Model file for the job. Use its own axes, mm. A direction names the side the tool comes from. Give positions to 0.01 mm unless a question says otherwise; leave off trailing zeros. Order: outer loops, then holes, each group sorted by start corner. A loop starts at its lowest first (then second) coordinate and runs counter-clockwise, first axis right, second up. Notation, with made-up numbers: (84, 30.25) -> (125, 30.25) arc R14 ccw to (125, 57.25) -> close; hole circle Ø3 at (58, 18). An arc over 180 degrees is marked (long way). Use CSV: the item, a comma, the result in double quotes. Start each with the question number.
1. Cut at B-B on z = 1.75. Give the number of separate pieces and of enclosed holes in the cut face, then the cut area to 3 significant figures.
2. Wall check: line 1 (X direction, y = 14.5, z = 11.5); line 2 (X direction, y = 1.25, z = -15.75); line 3 (X direction, y = 2.15, z = 19.75). Give the ranges that are in metal, low to high. Write a range as from..to.
3. Cut at C-C on z = 12.5. List the corners of the cut face in (x, y), then the cut area to 3 significant figures.
4. Drop flat-ended pins along their axis: pin 1 (18 mm diameter, centred on x = -1, z = 4.5, fed in from +Y); pin 2 (6 mm diameter, centred on y = 8, z = -17, fed in from +X); pin 3 (3 mm diameter, centred on y = 11.5, z = -7, fed in from -X); pin 4 (1 mm diameter, centred on x = -30.5, z = -3, fed in from -Y). Give the stop position or say it passes through.
5. Pull direction Z, two halves, no side cores. Call faces 4 (the flat face through (-70, 16, 0)), 5 (the cylindrical face through (-72.297, 6.535, -32.609)), 6 (the flat face through (16, 2, 8.25)): released by +Z, released by -Z, zero draft, split by the parting line, or undercut.
6. 3-axis set-ups, long thin cutter, end or side, ignore diameter. For faces 1 (the flat face through (-44.295, 2, 12)), 2 (the flat face through (-73.5, 9, 0)), 3 (the cylindrical face through (-73.609, 2.028, -33.797)): which of +Z, -Z, +X, -X, +Y, -Y reach the whole face in a straight line?
7. Cut at A-A on z = 19.75. List the corners of the cut face in (x, y).
```python
from build123d import *

# Parameters (mm, degrees)
SKETCH1_W           = 149.5
SKETCH1_H           = 70
BOSS_EXTRUDE1_DEPTH = 4
FILLET1_R           = 4
SKETCH6_W           = 147
SKETCH6_H           = 67.5
BOSS_EXTRUDE3_DEPTH = 5
FILLET2_R           = 4
SKETCH7_W           = 6.205469591
SKETCH7_H           = 30
BOSS_EXTRUDE4_DEPTH = 7
SKETCH8_R           = 1
CUT_EXTRUDE3_DEPTH  = 154.163515564
FILLET5_R           = 4
SKETCH9_W           = 134.589060818
SKETCH9_H           = 59.5
CUT_EXTRUDE4_DEPTH  = 5
FILLET7_R           = 2
SKETCH11_R          = 4
CUT_EXTRUDE5_DEPTH  = 84.406009975
SKETCH12_R          = 2.75
CUT_EXTRUDE6_DEPTH  = 84.406009975
SKETCH13_R          = 2.75
CUT_EXTRUDE7_DEPTH  = 84.406009975
SKETCH17_W          = 16
SKETCH17_H          = 13
CUT_EXTRUDE11_DEPTH = 84.406009975
SKETCH18_R          = 3
SKETCH18_W          = 15
SKETCH18_H          = 7
CUT_EXTRUDE12_DEPTH = 84.406009975
SKETCH19_W          = 6
SKETCH19_H          = 8
CUT_EXTRUDE13_DEPTH = 84.406009975
SKETCH20_R          = 1.5
CUT_EXTRUDE14_DEPTH = 84.406009975
SKETCH22_R          = 5.5
CUT_EXTRUDE15_DEPTH = 2
CHAMFER2_SIZE       = 2
SKETCH23_R          = 2.75
CUT_EXTRUDE16_DEPTH = 84.406009975
SKETCH24_R          = 5.1
CUT_EXTRUDE17_DEPTH = 2
CHAMFER3_SIZE       = 2


with BuildPart() as part:
    # Sketch1 → Boss-Extrude1 (new body)
    with BuildSketch(Plane(origin=(0, 0, 0), x_dir=(1, 0, 0), z_dir=(0, 1, 0))):
        Rectangle(SKETCH1_W, SKETCH1_H)
    extrude(amount=BOSS_EXTRUDE1_DEPTH)

    # Fillet1
    fillet1_edges = [part.edges().sort_by_distance(p)[0] for p in [
        (74.75, 2, 35),
        (-74.75, 2, 35),
        (-74.75, 2, -35),
        (74.75, 2, -35),
    ]]
    fillet(fillet1_edges, radius=FILLET1_R)

    # Sketch6 → Boss-Extrude3 (add)
    with BuildSketch(Plane(origin=(0, 4, 0), x_dir=(1, 0, 0), z_dir=(0, 1, 0))):
        Rectangle(SKETCH6_W, SKETCH6_H)
    extrude(amount=BOSS_EXTRUDE3_DEPTH)

    # Fillet2
    fillet2_edges = [part.edges().sort_by_distance(p)[0] for p in [
        (73.5, 6.5, 33.75),
        (73.5, 6.5, -33.75),
        (-73.5, 6.5, -33.75),
        (-73.5, 6.5, 33.75),
    ]]
    fillet(fillet2_edges, radius=FILLET2_R)

    # Sketch7 → Boss-Extrude4 (add)
    with BuildSketch(Plane(origin=(0, 9, 0), x_dir=(1, 0, 0), z_dir=(0, 1, 0))):
        with Locations((-70.397265205, 0)):
            Rectangle(SKETCH7_W, SKETCH7_H)
        with Locations((70.397265205, 0)):
            Rectangle(SKETCH7_W, SKETCH7_H)
    extrude(amount=BOSS_EXTRUDE4_DEPTH)

    # Sketch8 → Cut-Extrude3 (cut, through all)
    with BuildSketch(Plane.ZY.offset(73.5)):
        with Locations((-7, 11.5)):
            Circle(SKETCH8_R)
        with Locations((7, 11.5)):
            Circle(SKETCH8_R)
    extrude(amount=-CUT_EXTRUDE3_DEPTH, mode=Mode.SUBTRACT)

    # Fillet5
    fillet5_edges = [part.edges().sort_by_distance(p)[0] for p in [
        (-70.397265204, 16, 15),
        (-70.397265204, 16, -15),
        (70.397265204, 16, -15),
        (70.397265204, 16, 15),
    ]]
    fillet(fillet5_edges, radius=FILLET5_R)

    # Sketch9 → Cut-Extrude4 (cut)
    with BuildSketch(Plane(origin=(0, 9, 0), x_dir=(1, 0, 0), z_dir=(0, 1, 0))):
        Rectangle(SKETCH9_W, SKETCH9_H)
    extrude(amount=-CUT_EXTRUDE4_DEPTH, mode=Mode.SUBTRACT)

    # Fillet7
    fillet7_edges = [part.edges().sort_by_distance(p)[0] for p in [
        (67.294530409, 6.5, -29.75),
        (67.294530409, 6.5, 29.75),
        (-67.294530409, 6.5, 29.75),
        (-67.294530409, 6.5, -29.75),
    ]]
    fillet(fillet7_edges, radius=FILLET7_R)

    # Sketch11 → Cut-Extrude5 (cut, through all)
    with BuildSketch(Plane(origin=(0, 4, 0), x_dir=(1, 0, 0), z_dir=(0, 1, 0))):
        with Locations(Location((57.294530409, -19.75, 0), (0, 0, 270))):
            Circle(SKETCH11_R)
    extrude(amount=-CUT_EXTRUDE5_DEPTH, mode=Mode.SUBTRACT)

    # Sketch12 → Cut-Extrude6 (cut, through all)
    with BuildSketch(Plane(origin=(0, 4, 0), x_dir=(1, 0, 0), z_dir=(0, 1, 0))):
        with Locations(Location((57.294530409, -1.75, 0), (0, 0, 270))):
            Circle(SKETCH12_R)
    extrude(amount=-CUT_EXTRUDE6_DEPTH, mode=Mode.SUBTRACT)

    # Sketch13 → Cut-Extrude7 (cut, through all)
    with BuildSketch(Plane(origin=(0, 4, 0), x_dir=(1, 0, 0), z_dir=(0, 1, 0))):
        with Locations(Location((57.294530409, 15.75, 0), (0, 0, 270))):
            Circle(SKETCH13_R)
    extrude(amount=-CUT_EXTRUDE7_DEPTH, mode=Mode.SUBTRACT)

    # Sketch17 → Cut-Extrude11 (cut, through all)
    with BuildSketch(Plane(origin=(0, 4, 0), x_dir=(1, 0, 0), z_dir=(0, 1, 0))):
        with Locations((-47.294530409, 16.75)):
            Rectangle(SKETCH17_W, SKETCH17_H)
    extrude(amount=-CUT_EXTRUDE11_DEPTH, mode=Mode.SUBTRACT)

    # Sketch18 → Cut-Extrude12 (cut, through all)
    with BuildSketch(Plane(origin=(0, 4, 0), x_dir=(1, 0, 0), z_dir=(0, 1, 0))):
        with Locations(Location((-41.294530409, -11.75, 0), (0, 0, 270))):
            Circle(SKETCH18_R)
        with Locations(Location((-54.794530409, -11.75, 0), (0, 0, 270))):
            Circle(SKETCH18_R)
        with Locations((15.705469591, -11.75)):
            Rectangle(SKETCH18_W, SKETCH18_H)
        with Locations((-10.794530409, -11.75)):
            Rectangle(SKETCH18_W, SKETCH18_H)
    extrude(amount=-CUT_EXTRUDE12_DEPTH, mode=Mode.SUBTRACT)

    # Sketch19 → Cut-Extrude13 (cut, through all)
    with BuildSketch(Plane(origin=(0, 4, 0), x_dir=(1, 0, 0), z_dir=(0, 1, 0))):
        with Locations((-41.294530409, -11.75)):
            Rectangle(SKETCH19_W, SKETCH19_H)
        with Locations((-54.794530409, -11.75)):
            Rectangle(SKETCH19_W, SKETCH19_H)
    extrude(amount=-CUT_EXTRUDE13_DEPTH, mode=Mode.SUBTRACT)

    # Sketch20 → Cut-Extrude14 (cut, through all)
    with BuildSketch(Plane(origin=(0, 4, 0), x_dir=(1, 0, 0), z_dir=(0, 1, 0))):
        with Locations(Location((-60.794530409, 16.75, 0), (0, 0, 270))):
            Circle(SKETCH20_R)
        with Locations(Location((-33.794530409, 16.75, 0), (0, 0, 90))):
            Circle(SKETCH20_R)
    extrude(amount=-CUT_EXTRUDE14_DEPTH, mode=Mode.SUBTRACT)

    # Sketch22 → Cut-Extrude15 (cut)
    with BuildSketch(Plane(origin=(0, 4, 0), x_dir=(1, 0, 0), z_dir=(0, 1, 0))):
        with Locations(Location((57.294530409, 15.75, 0), (0, 0, 270))):
            Circle(SKETCH22_R)
    extrude(amount=-CUT_EXTRUDE15_DEPTH, mode=Mode.SUBTRACT)

    # Chamfer2
    chamfer2_edges = [part.edges().sort_by_distance(p)[0] for p in [
        (57.294530409, 4, -21.25),
    ]]
    chamfer(chamfer2_edges, length=CHAMFER2_SIZE - 0.0001)  # a hair under: the kernel refuses the full size

    # Sketch23 → Cut-Extrude16 (cut, through all)
    with BuildSketch(Plane(origin=(0, 4, 0), x_dir=(1, 0, 0), z_dir=(0, 1, 0))):
        with Locations(Location((41.294530409, -1.75, 0), (0, 0, 270))):
            Circle(SKETCH23_R)
    extrude(amount=-CUT_EXTRUDE16_DEPTH, mode=Mode.SUBTRACT)

    # Sketch24 → Cut-Extrude17 (cut)
    with BuildSketch(Plane(origin=(0, 4, 0), x_dir=(1, 0, 0), z_dir=(0, 1, 0))):
        with Locations(Location((41.294530409, -1.75, 0), (0, 0, 270))):
            Circle(SKETCH24_R)
    extrude(amount=-CUT_EXTRUDE17_DEPTH, mode=Mode.SUBTRACT)

    # Chamfer3
    chamfer3_edges = [part.edges().sort_by_distance(p)[0] for p in [
        (41.294530409, 4, -3.35),
    ]]
    chamfer(chamfer3_edges, length=CHAMFER3_SIZE - 0.0001)  # a hair under: the kernel refuses the full size


solid = part.part
```
Verdict:
1,separate pieces,"3"
1,enclosed holes,"0"
1,area,"690 mm^2"
2,line 1,"-73.5..-67.29, 67.29..73.5"
2,line 2,"-74.75..-61.91, -59.68..-55.29, -39.29..-34.91, -32.68..54.54, 60.04..74.75"
2,line 3,"-74.75..53.29, 61.29..74.75"
3,outline,"(-74.75, 0) -> (-57.79, 0) -> (-57.79, 4) -> (-67.29, 4) -> (-67.29, 15.71) -> (-73.5, 15.71) -> (-73.5, 4) -> (-74.75, 4) -> close; (-51.79, 0) -> (-44.29, 0) -> (-44.29, 4) -> (-51.79, 4) -> close; (-38.29, 0) -> (-18.29, 0) -> (-18.29, 4) -> (-38.29, 4) -> close; (-3.29, 0) -> (8.21, 0) -> (8.21, 4) -> (-3.29, 4) -> close; (23.21, 0) -> (74.75, 0) -> (74.75, 4) -> (73.5, 4) -> (73.5, 15.71) -> (67.29, 15.71) -> (67.29, 4) -> (23.21, 4) -> close"
3,area,"575 mm^2"
4,pin 1,"y = 4"
4,pin 2,"x = 73.5"
4,pin 3,"x = -73.5"
4,pin 4,"y = 0"
5,face 4,"zero draft"
5,face 5,"released by -Z"
5,face 6,"undercut"
6,face 1,"+Y, -Y"
6,face 2,"+Z, -Z, -X, +Y"
6,face 3,"-Z, -X, +Y, -Y"
7,outline,"(-74.75, 0) -> (53.29, 0) -> (53.29, 4) -> (-67.29, 4) -> (-67.29, 9) -> (-73.5, 9) -> (-73.5, 4) -> (-74.75, 4) -> close; (61.29, 0) -> (74.75, 0) -> (74.75, 4) -> (73.5, 4) -> (73.5, 9) -> (67.29, 9) -> (67.29, 4) -> (61.29, 4) -> close"
